from build123d import *

# Parameters (mm, degrees)
BOSS_EXTRUDE1_DEPTH      = 20
BOSS_EXTRUDE1_DEPTH_BACK = 4
SKETCH1_R                = 6.3
SKETCH2_W                = 40
SKETCH2_H                = 3.045079522
CUT_EXTRUDE1_DEPTH       = 10


with BuildPart() as part:
    # Sketch1 → Boss-Extrude1 (new, two sides: drawn at the far end of the back side and taken through both)
    with BuildSketch(Plane.XY.offset(-BOSS_EXTRUDE1_DEPTH_BACK)):
        with BuildLine():
            ThreePointArc((-44.914648696, 10), (-47.601146738, 9.216957229), (-49.446187631, 7.113091309))
            Line((-49.446187631, 7.113091309), (-72.088476723, -41.443454346))
            ThreePointArc((-72.088476723, -41.443454346), (-71.93118587, -43.843249021), (-69.822707256, -45))
            Line((-69.822707256, -45), (41.247707256, -45))
            ThreePointArc((41.247707256, -45), (43.35618587, -43.843249021), (43.513476723, -41.443454346))
            Line((43.513476723, -41.443454346), (20.871187631, 7.113091309))
            ThreePointArc((20.871187631, 7.113091309), (19.026146738, 9.216957229), (16.339648696, 10))
            Line((16.339648696, 10), (-44.914648696, 10))
        make_face()
        with Locations((9.525, 0)):
            Circle(SKETCH1_R, mode=Mode.SUBTRACT)
        with Locations((-38.1, 0)):
            Circle(SKETCH1_R, mode=Mode.SUBTRACT)
    extrude(amount=BOSS_EXTRUDE1_DEPTH + BOSS_EXTRUDE1_DEPTH_BACK)

    # Sketch2 → Cut-Extrude1 (cut)
    with BuildSketch(Plane.XY.offset(20)):
        with Locations((4.975032248, -34.522539761)):
            Rectangle(SKETCH2_W, SKETCH2_H)
    extrude(amount=-CUT_EXTRUDE1_DEPTH, mode=Mode.SUBTRACT)


solid = part.part
Read the model definition and answer for the solid it produces. Units are mm, in the model's axes. A direction names the side the tool comes from. Round coordinates to 2 decimals unless told otherwise and drop trailing zeros. Loops run counter-clockwise (first coordinate to the right, second up) from the corner with the lowest first, then second, coordinate; pieces in that order, holes last.
Q1. Which of the six approach directions +Z, -Z, +X, -X, +Y, -Y give full straight-line access (tool end or side, diameter ignored) to faces 1 (the face through (-15.025, -35, 15)), 2 (the face through (19.06, 9.195, 7.832))?
Q2. Consider probe 1 along Y at (x, z) = (-38.1, 10.25); probe 2 along X at (y, z) = (2.5, 13.5); probe 3 along Y at (x, z) = (11, 17.5). Determine where each line is inside the solid, lowest interval first.
Q3. Section B-B on z = 2.25 is taken. Write down the section's boundary in (x, y) (3 decimals).
Q4. Section C-C on y = -3 is taken. Write down the section's boundary in (x, z).
Q5. Section A-A on x = -38.1 is taken. Write down the section's boundary in (y, z), and give its area (3 significant figures).
Q6. Each of these flat-tipped pins is pushed along its axis until it touches: pin 1 (4 mm diameter, centred on y = -18, z = 5.5, fed in from -X); pin 2 (10 mm diameter, centred on y = -21, z = 11, fed in from +X); pin 3 (6 mm diameter, centred on y = -3.5, z = 7.5, fed in from -X). Where does it stop, or does it pass through?
Q7. Determine the mould class of faces 3 (the face through (-44.394, 0.277, 7.832)), 4 (the face through (5, -33, 15)), 5 (the face through (-15, -45, 8)), 6 (the face through (-15, -17, 20)) for opening direction Y: released by +Y, released by -Y, zero draft, split by the parting line, or undercut.
Q8. Section D-D on x = 1.5 is taken. Write down the section's boundary in (y, z).
Output:
1. face 1: +Z
1. face 2: +Z, -Z, +X, +Y
2. probe 1: y = -45 to -6.3, 6.3 to 10
2. probe 2: x = -51.6 to -43.88, -32.32 to 3.74, 15.31 to 23.02
2. probe 3: y = -45 to -36.05, -33 to -6.12, 6.12 to 10
3. outline: (-72.088, -41.443) arc R2.5 ccw to (-69.823, -45) - (41.248, -45) arc R2.5 ccw to (43.513, -41.443) - (20.871, 7.113) arc R5 ccw to (16.34, 10) - (-44.915, 10) arc R5 ccw to (-49.446, 7.113) - close; hole circle Ø12.6 at (-38.1, 0); hole circle Ø12.6 at (9.525, 0)
4. outline: (-54.16, -4) - (-43.64, -4) - (-43.64, 20) - (-54.16, 20) - close; (-32.56, -4) - (3.99, -4) - (3.99, 20) - (-32.56, 20) - close; (15.06, -4) - (25.59, -4) - (25.59, 20) - (15.06, 20) - close
5. outline: (-45, -4) - (-6.3, -4) - (-6.3, 20) - (-45, 20) - close; (6.3, -4) - (10, -4) - (10, 20) - (6.3, 20) - close
5. area: 1,020 mm2
6. pin 1: stops at x = -62.09
6. pin 2: stops at x = 36.31
6. pin 3: stops at x = -55.79
7. face 3: undercut
7. face 4: undercut
7. face 5: released by -Y
7. face 6: zero draft
8. outline: (-45, -4) - (10, -4) - (10, 20) - (-33, 20) - (-33, 10) - (-36.05, 10) - (-36.05, 20) - (-45, 20) - close
